Answer from the drawing. Dimensions are ordinates in mm from the lowest x, y and z of the part. Coordinates: 2 decimals unless noted, no trailing zeros. Loops run counter-clockwise (first coordinate to the right, second up) from the corner with the lowest first, then second, coordinate; pieces in that order, holes last. Notation, with made-up numbers: M 1,63 L 52,63 A20 ccw 52,102 Z; hole C -22.5,54 d4. An arc over 180 degrees is marked long. Put each result on its own line as item: value.
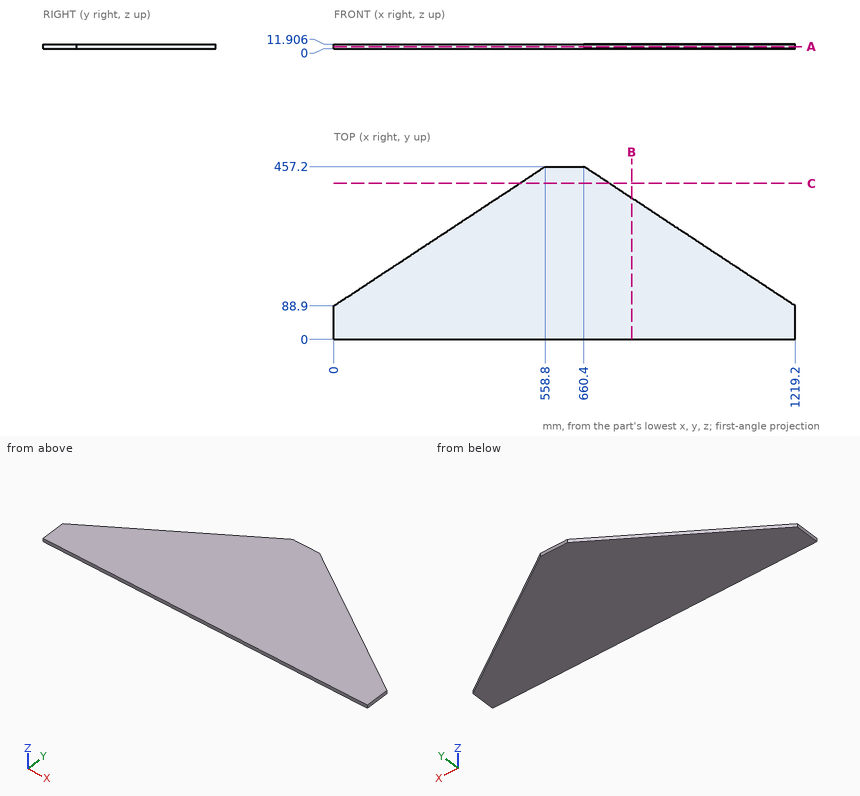
1) Find section B-B, the plane x = 787. Write down the section's boundary in (y, z), plus the area to 3 significant figures.
Answer list:
outline: M 0,0 L 373.76,0 L 373.76,11.91 L 0,11.91 Z
area: 4,450 mm^2
2) Find section A-A, the plane z = 4.75. Write down the section's boundary in (x, y).
Answer list:
outline: M 0,0 L 1219.2,0 L 1219.2,88.9 L 660.4,457.2 L 558.8,457.2 L 0,88.9 Z
3) Given pin 1 Ø2 at (y, z) = (189.5, 10) entering from -X; pin 2 Ø2 at (y, z) = (375.5, 7) entering from -X (1 decimal); pin 3 Ø6 at (x, z) = (876.5, 8.5) entering from -Y; pin 4 Ø3 at (y, z) = (409, 8.5) entering from -X, each flat-ended and moving along its own axis, determine where each tip first touches the part or whether it passes through.
Answer list:
pin 1: stops at x = 151.12
pin 2: stops at x = 433.3
pin 3: stops at y = 0
pin 4: stops at x = 483.39
4) Straight lines are drawn through the part: line 1 (Y direction, x = 288, z = 10.25); line 2 (X direction, y = 131, z = 1.75) (1 decimal); line 3 (Y direction, x = 1054.5, z = 3.5). For each, find the intervals that lie inside material, in ascending order. Write a range as [from, to].
Answer list:
line 1: y = [0, 278.72]
line 2: x = [63.9, 1155.3]
line 3: y = [0, 197.45]
5) Find section C-C, the plane y = 412.5. Write down the section's boundary in (x, z), plus the area to 3 significant figures.
Answer list:
outline: M 490.98,0 L 728.22,0 L 728.22,11.91 L 490.98,11.91 Z
area: 2,820 mm^2
